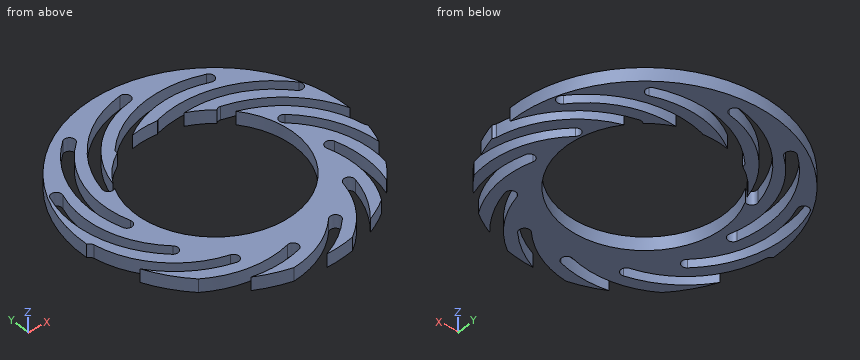
from build123d import *

# Parameters (mm, degrees)
SKETCH4_R           = 5
SKETCH4_R_2         = 3
BOSS_EXTRUDE2_DEPTH = 0.5
CUT_EXTRUDE1_DEPTH  = 0.5


with BuildPart() as part:
    # Sketch4 → Boss-Extrude2 (new body)
    with BuildSketch(Plane.XY):
        Circle(SKETCH4_R)
        Circle(SKETCH4_R_2, mode=Mode.SUBTRACT)
    extrude(amount=BOSS_EXTRUDE2_DEPTH)

    # Sketch5 → Cut-Extrude1 (cut)
    with BuildSketch(Plane.XY):
        with BuildLine():
            ThreePointArc((2.838380277, 3.735395811), (0.523052201, 3.89223631), (-1.488789119, 2.735587034))
            ThreePointArc((-1.488789119, 2.735587034), (-1.479999142, 2.452880939), (-1.197293047, 2.461670915))
            ThreePointArc((-1.197293047, 2.461670915), (0.613101285, 3.502504142), (2.696594047, 3.361368186))
            ThreePointArc((2.696594047, 3.361368186), (2.954500975, 3.477488883), (2.838380277, 3.735395811))
        make_face()
        with BuildLine():
            ThreePointArc((4.336939093, 1.463159243), (2.603149411, 2.627132948), (0.514885315, 2.630942098))
            ThreePointArc((0.514885315, 2.630942098), (0.265659666, 2.764682803), (0.399400371, 3.013908452))
            ThreePointArc((0.399400371, 3.013908452), (2.7200307, 3.009675448), (4.646743383, 1.716183554))
            ThreePointArc((4.646743383, 1.716183554), (4.618353394, 1.434769253), (4.336939093, 1.463159243))
        make_face()
        with BuildLine():
            ThreePointArc((4.808415103, -1.000910445), (3.888896046, 0.874015193), (2.082310864, 1.921446063))
            ThreePointArc((2.082310864, 1.921446063), (1.933345473, 2.161881735), (2.173781146, 2.310847125))
            ThreePointArc((2.173781146, 2.310847125), (4.181389462, 1.146866072), (5.203225644, -0.93668711))
            ThreePointArc((5.203225644, -0.93668711), (5.037932041, -1.166204048), (4.808415103, -1.000910445))
        make_face()
        with BuildLine():
            ThreePointArc((3.98469046, -3.370595397), (4.125826417, -1.287102636), (3.08499319, 0.523291697))
            ThreePointArc((3.08499319, 0.523291697), (3.076203214, 0.805997792), (3.358909309, 0.814787769))
            ThreePointArc((3.358909309, 0.814787769), (4.515558585, -1.197053551), (4.358718086, -3.512381628))
            ThreePointArc((4.358718086, -3.512381628), (4.100811158, -3.628502325), (3.98469046, -3.370595397))
        make_face()
        with BuildLine():
            ThreePointArc((2.086481518, -5.010940443), (3.250455223, -3.277150761), (3.254264373, -1.188886665))
            ThreePointArc((3.254264373, -1.188886665), (3.388005078, -0.939661016), (3.637230727, -1.073401721))
            ThreePointArc((3.637230727, -1.073401721), (3.632997723, -3.394032051), (2.339505829, -5.320744734))
            ThreePointArc((2.339505829, -5.320744734), (2.058091528, -5.292354744), (2.086481518, -5.010940443))
        make_face()
        with BuildLine():
            ThreePointArc((-0.37758817, -5.482416453), (1.497337468, -4.562897396), (2.544768337, -2.756312214))
            ThreePointArc((2.544768337, -2.756312214), (2.78520401, -2.607346824), (2.9341694, -2.847782496))
            ThreePointArc((2.9341694, -2.847782496), (1.770188347, -4.855390812), (-0.313364835, -5.877226994))
            ThreePointArc((-0.313364835, -5.877226994), (-0.542881773, -5.711933391), (-0.37758817, -5.482416453))
        make_face()
        with BuildLine():
            ThreePointArc((-2.747273122, -4.658691811), (-0.663780361, -4.799827767), (1.146613972, -3.75899454))
            ThreePointArc((1.146613972, -3.75899454), (1.429320067, -3.750204564), (1.438110043, -4.032910659))
            ThreePointArc((1.438110043, -4.032910659), (-0.573731276, -5.189559935), (-2.889059353, -5.032719436))
            ThreePointArc((-2.889059353, -5.032719436), (-3.00518005, -4.774812508), (-2.747273122, -4.658691811))
        make_face()
        with BuildLine():
            ThreePointArc((-4.387618168, -2.760482868), (-2.653828487, -3.924456573), (-0.56556439, -3.928265723))
            ThreePointArc((-0.56556439, -3.928265723), (-0.316338742, -4.062006428), (-0.450079446, -4.311232077))
            ThreePointArc((-0.450079446, -4.311232077), (-2.770709776, -4.306999073), (-4.697422459, -3.013507179))
            ThreePointArc((-4.697422459, -3.013507179), (-4.669032469, -2.732092879), (-4.387618168, -2.760482868))
        make_face()
        with BuildLine():
            ThreePointArc((-4.859094178, -0.29641318), (-3.939575121, -2.171338818), (-2.132989939, -3.218769688))
            ThreePointArc((-2.132989939, -3.218769688), (-1.984024549, -3.45920536), (-2.224460221, -3.60817075))
            ThreePointArc((-2.224460221, -3.60817075), (-4.232068537, -2.444189697), (-5.253904719, -0.360636515))
            ThreePointArc((-5.253904719, -0.360636515), (-5.088611116, -0.131119577), (-4.859094178, -0.29641318))
        make_face()
        with BuildLine():
            ThreePointArc((-4.035369536, 2.073271772), (-4.176505492, -0.01022099), (-3.135672265, -1.820615322))
            ThreePointArc((-3.135672265, -1.820615322), (-3.126882289, -2.103321417), (-3.409588384, -2.112111394))
            ThreePointArc((-3.409588384, -2.112111394), (-4.56623766, -0.100270074), (-4.409397161, 2.215058003))
            ThreePointArc((-4.409397161, 2.215058003), (-4.151490233, 2.3311787), (-4.035369536, 2.073271772))
        make_face()
        with BuildLine():
            ThreePointArc((-2.137160594, 3.713616818), (-3.301134298, 1.979827136), (-3.304943449, -0.10843696))
            ThreePointArc((-3.304943449, -0.10843696), (-3.438684153, -0.357662609), (-3.687909802, -0.223921904))
            ThreePointArc((-3.687909802, -0.223921904), (-3.683676798, 2.096708426), (-2.390184904, 4.023421109))
            ThreePointArc((-2.390184904, 4.023421109), (-2.108770604, 3.995031119), (-2.137160594, 3.713616818))
        make_face()
        with BuildLine():
            ThreePointArc((0.326909095, 4.185092828), (-1.548016544, 3.265573771), (-2.595447413, 1.458988589))
            ThreePointArc((-2.595447413, 1.458988589), (-2.835883085, 1.310023199), (-2.984848475, 1.550458871))
            ThreePointArc((-2.984848475, 1.550458871), (-1.820867422, 3.558067187), (0.26268576, 4.579903369))
            ThreePointArc((0.26268576, 4.579903369), (0.492202698, 4.414609766), (0.326909095, 4.185092828))
        make_face()
    extrude(amount=CUT_EXTRUDE1_DEPTH, mode=Mode.SUBTRACT)


solid = part.part
Can you work these out from the model? Positions are in its coordinate system, mm. Coordinates: 2 decimals unless noted, no trailing zeros. Write each loop counter-clockwise with the first axis right and the second up, starting at its lowest first coordinate (ties: lowest second). Pieces come first, ordered by that corner, then holes. Notation, with made-up numbers: (77, 27.25) - (103, 27.25) arc R24 cw to (103, 65.25) - close; hole circle Ø3 at (9.25, 53.25). An arc over 180 degrees is marked (long way). Return JSON: item names as keys, results as strings. Group by question number.
Item 1: If we section it at A-A (x = -1): Write out the boundary of the cut face in (y, z), then the cut area to 3 significant figures.
Item 2: I'm going to push a flat-ended pin straight in: pin 1 Ø1 at (x, y) = (2, 0.5) entering from +Z. Where does the tip first touch, or does it pass through?
Item 3: If we section it at B-B (z = 0.1): Count the separate pieces of the cut face and the enclosed holes in it, then the cut area to 3 significant figures.
Item 4: Please list where these lines run through material, in increasing order: probe 1 along X at (y, z) = (2.5, 0.3); probe 2 along X at (y, z) = (-0.5, 0.4); probe 3 along X at (y, z) = (-1, 0.05).
Return value:
{
 "1": {"outline": "(-4.86, 0) - (-4.44, 0) - (-4.44, 0.5) - (-4.86, 0.5) - close; (-4.03, 0) - (-2.83, 0) - (-2.83, 0.5) - (-4.03, 0.5) - close; (3.18, 0) - (3.69, 0) - (3.69, 0.5) - (3.18, 0.5) - close; (4.15, 0) - (4.9, 0) - (4.9, 0.5) - (4.15, 0.5) - close", "area": "1.44 mm^2"},
 "2": {"pin 1": "passes through"},
 "3": {"separate pieces": "1", "enclosed holes": "2", "area": "32.3 mm^2"},
 "4": {"probe 1": "x = -4.33 to -3.54, -3.1 to -2.63, -2.17 to -1.66, 1.66 to 2.95, 3.79 to 4.33", "probe 2": "x = -4.82 to -4.45, -4.03 to -2.96, 2.96 to 3.84, 4.29 to 4.69", "probe 3": "x = -4.67 to -4.24, -3.79 to -2.83, 2.83 to 3.29, 3.6 to 4.05, 4.46 to 4.81"}
}
